Read the model definition and answer for the solid it produces. Units are mm, in the model's axes. A direction names the side the tool comes from. Coordinates: 2 decimals unless noted, no trailing zeros. Write each loop counter-clockwise with the first axis right and the second up, starting at its lowest first coordinate (ties: lowest second). Pieces come first, ordered by that corner, then holes.
1) Each of these flat-tipped pins is pushed along its axis until it touches: pin 1 Ø1.5 at (x, z) = (-17.5, -6) entering from +Y; pin 2 Ø4.5 at (x, z) = (0, -8) entering from +Y; pin 3 Ø2.5 at (x, z) = (17.5, -7) entering from +Y. Where does it stop, or does it pass through?
2) The part is cut by section C-C (z = -2). Give the number of separate pieces and of enclosed holes in the cut face, then the cut area to 3 significant figures.
3) The part is cut by section A-A (x = 0). Determine the outline of the cut face in (y, z).
4) Determine the mould class of faces 6 (the face through (-0.39, 2.653, -9.757)), 7 (the face through (-14.85, -8, -2)), 8 (the face through (17, 2.16, -5)), 9 (the face through (-19.85, 0, 1)) for opening direction X: +X half, -X half, draft (parallel to the pull), parting line (faces both ways), or undercut.
5) The part is cut by section D-D (x = 8.5). Determine the outline of the cut face in (y, z).
6) Find the intervals of material crossed by line 1 (Z direction, x = 0, y = 3); line 2 (Y direction, x = 3, z = -10); line 3 (Z direction, x = 1, y = -28.5), in increasing order.
7) The part is cut by section B-B (y = 1.5). Determine the outline of the cut face in (x, z), then the cut area to 3 significant figures.
8) Which of the six approach directions +Z, -Z, +X, -X, +Y, -Y give full straight-line access (tool end or side, diameter ignored) to faces 1 (the face through (0, 32.5, 1)), 2 (the face through (0, 0, 0)), 3 (the face through (0, 3.16, -5)), 4 (the face through (0, -2.16, -6)), 5 (the face through (14.85, 8, -2))?
from build123d import *

# Parameters (mm, degrees)
F0_W             = 39.7
F0_H             = 65
F1_DEPTH         = 2
F3_DEPTH         = 5
F3_COPIES2_COUNT = 2
F5_DEPTH         = 5
F6_R             = 1.8
F7_DEPTH         = 35.6610001


# Not quite as in the source:
# - a pattern or mirror of a feature is missing from the dataset's text; its kind, count and spacing are read off the source's solid


with BuildPart() as f1:
    # F0 (on Top) → F1 (new body)
    with BuildSketch(Plane.XY):
        Rectangle(F0_W, F0_H)
    extrude(amount=F1_DEPTH)

    # F2 (on face) → F3 (join)
    with BuildSketch(Plane.YZ.offset(19.85)):
        with BuildLine():
            add(Edge.make_bspline(
                [(-2.16, -10), (-2.16, 0), (-32.5, 0)],
                knots=[0, 0, 0, 1.5707963268, 1.5707963268, 1.5707963268], degree=2, weights=[1, 0.7071067812, 1]))
            Line((-2.16, -10), (-2.16, 0))
            Line((-2.16, 0), (-32.5, 0))
        make_face()
    f3 = extrude(amount=-F3_DEPTH)

    # F3_copies: F3 across plane
    add(f3.mirror(Plane.ZX))

    # F3_copies1: F3 across plane
    add(f3.mirror(Plane(origin=(0, 0, 0), x_dir=(0, 0, -1), z_dir=(-1, 0, 0))))

    # F3_copies2: F3 ×2 about axis
    f3_copies2_axis = Axis((0, 0, 0), (0, 0, 1))
    for i in range(1, F3_COPIES2_COUNT):
        add(f3.rotate(f3_copies2_axis, i * 360 / F3_COPIES2_COUNT))

    # F4 (on Right) → F5 (join, symmetric)
    with BuildSketch(Plane.YZ):
        Polygon((-2.16, -14), (-2.16, -10), (-2.16, 0), (-3.16, 0), (-3.16, -14), align=None)
    f5 = extrude(amount=F5_DEPTH, both=True)

    # F5_copies: F5 across plane
    add(f5.mirror(Plane.ZX))

    # F6 (on face) → F7 (cut, through all)
    with BuildSketch(Plane.XZ.offset(3.16)):
        with Locations((0, -8)):
            Circle(F6_R)
    extrude(amount=-F7_DEPTH, mode=Mode.SUBTRACT)


solid = f1.part
Reported:
1. pin 1: stops at y = 5.8
1. pin 2: stops at y = 3.16
1. pin 3: stops at y = 5.04
2. separate pieces: 6
2. enclosed holes: 0
2. area: 263 mm2
3. outline: (-32.5, 0) - (-3.16, 0) - (-3.16, -6.2) - (-2.16, -6.2) - (-2.16, 0) - (2.16, 0) - (2.16, -6.2) - (3.16, -6.2) - (3.16, 0) - (32.5, 0) - (32.5, 2) - (-32.5, 2) - close; (-3.16, -14) - (-2.16, -14) - (-2.16, -9.8) - (-3.16, -9.8) - close; (2.16, -14) - (3.16, -14) - (3.16, -9.8) - (2.16, -9.8) - close
4. face 6: undercut
4. face 7: undercut
4. face 8: draft
4. face 9: -X half
5. outline: (-32.5, 0) - (32.5, 0) - (32.5, 2) - (-32.5, 2) - close
6. line 1: z = -14 to -9.8, -6.2 to 2
6. line 2: y = -3.16 to -2.16, 2.16 to 3.16
6. line 3: z = 0 to 2
7. outline: (-19.85, 0) - (19.85, 0) - (19.85, 2) - (-19.85, 2) - close
7. area: 79.4 mm2
8. face 1: +Z, -Z, +X, -X, +Y
8. face 2: -Z
8. face 3: -Z, +Y
8. face 4: -Z, +X, -X
8. face 5: -Z, +Y, -Y
